```python
from build123d import *

# Parameters (mm, degrees)
SKETCH1_W                                        = 160
SKETCH1_H                                        = 150
BOSS_EXTRUDE1_DEPTH                              = 4.76
F_7_0_7_DIAMETER_HOLE1_D                         = 7
CBORE_FOR_M3_HEX_HEAD_MACHINE_SCREW1_D           = 3.5
CBORE_FOR_M3_HEX_HEAD_MACHINE_SCREW1_CBORE_D     = 6.5
CBORE_FOR_M3_HEX_HEAD_MACHINE_SCREW1_CBORE_DEPTH = 2
F_3_0_3_DIAMETER_HOLE1_D                         = 3
M27_CLEARANCE_HOLE1_D                            = 30


with BuildPart() as part:
    # Sketch1 → Boss-Extrude1 (new body)
    with BuildSketch(Plane.XY.offset(4.76)):
        with Locations((-10, 0)):
            Rectangle(SKETCH1_W, SKETCH1_H)
    extrude(amount=-BOSS_EXTRUDE1_DEPTH)

    # Sketch2 → Cut-Revolve1 (revolve, cut)
    with BuildSketch(Plane(origin=(0, 36.935244785, 0), x_dir=(1, 0, 0), z_dir=(0, 1, 0))):
        Polygon((35.647279442, 0), (34.026279442, 0), (34.026279442, -4.76), (35.647279442, -4.76), (35.647279442, -2.76), align=None)
    revolve(axis=Axis((34.026279442, 36.935244785, 0), (0, 0, 1)), mode=Mode.SUBTRACT)

    # Sketch3 → Cut-Revolve2 (revolve, cut)
    with BuildSketch(Plane(origin=(0, 11, 0), x_dir=(1, 0, 0), z_dir=(0, 1, 0))):
        Polygon((-47.379, 0), (-49, 0), (-49, -4.76), (-47.379, -4.76), (-47.379, -2.76), align=None)
    revolve(axis=Axis((-49, 11, 0), (0, 0, 1)), mode=Mode.SUBTRACT)

    # Sketch4 → Cut-Revolve3 (revolve, cut)
    with BuildSketch(Plane(origin=(0, -36.935244785, 0), x_dir=(1, 0, 0), z_dir=(0, 1, 0))):
        Polygon((35.647279442, 0), (34.026279442, 0), (34.026279442, -4.76), (35.647279442, -4.76), (35.647279442, -2.76), align=None)
    revolve(axis=Axis((34.026279442, -36.935244785, 0), (0, 0, 1)), mode=Mode.SUBTRACT)

    # Sketch5 → Cut-Revolve4 (revolve, cut)
    with BuildSketch(Plane(origin=(0, -47.935244785, 0), x_dir=(1, 0, 0), z_dir=(0, 1, 0))):
        Polygon((16.594720558, 0), (14.973720558, 0), (14.973720558, -4.76), (16.594720558, -4.76), (16.594720558, -2.76), align=None)
    revolve(axis=Axis((14.973720558, -47.935244785, 0), (0, 0, 1)), mode=Mode.SUBTRACT)

    # Sketch6 → Cut-Revolve5 (revolve, cut)
    with BuildSketch(Plane(origin=(0, 47.935244785, 0), x_dir=(1, 0, 0), z_dir=(0, 1, 0))):
        Polygon((16.594720558, 0), (14.973720558, 0), (14.973720558, -4.76), (16.594720558, -4.76), (16.594720558, -2.76), align=None)
    revolve(axis=Axis((14.973720558, 47.935244785, 0), (0, 0, 1)), mode=Mode.SUBTRACT)

    # Sketch7 → Cut-Revolve6 (revolve, cut)
    with BuildSketch(Plane(origin=(0, -11, 0), x_dir=(1, 0, 0), z_dir=(0, 1, 0))):
        Polygon((-47.379, 0), (-49, 0), (-49, -4.76), (-47.379, -4.76), (-47.379, -2.76), align=None)
    revolve(axis=Axis((-49, -11, 0), (0, 0, 1)), mode=Mode.SUBTRACT)

    # Ø7.0 (7) Diameter Hole1 (through all)
    with Locations(Plane(origin=(0, 0, 0), x_dir=(-1, 0, 0), z_dir=(0, 0, -1))):
        with Locations((3, -41.5)):
            Hole(F_7_0_7_DIAMETER_HOLE1_D / 2)

    # CBORE for M3 Hex Head Machine Screw1 (through all)
    with Locations(Plane.XY.offset(4.76)):
        with Locations((-70, -70), (60, -60), (-84.999999999, 54.667182961), (60, 54.667182961), (-84.999999999, -38.000000001)):
            CounterBoreHole(CBORE_FOR_M3_HEX_HEAD_MACHINE_SCREW1_D / 2, CBORE_FOR_M3_HEX_HEAD_MACHINE_SCREW1_CBORE_D / 2, CBORE_FOR_M3_HEX_HEAD_MACHINE_SCREW1_CBORE_DEPTH)

    # Ø3.0 (3) Diameter Hole1 (through all)
    with Locations(Plane(origin=(0, 0, 0), x_dir=(-1, 0, 0), z_dir=(0, 0, -1))):
        with Locations((20.75, 35.940054257), (18.25, 31.609927238), (20.75, -35.940054257), (18.25, -31.609927238), (-41.5, 0), (-29.250000001, 50.662486121), (-26.750000001, 46.332359102), (-36.5, 0), (58.5, 1e-09), (53.5, 1e-09), (-26.749999999, -46.332359103), (-29.249999999, -50.662486122)):
            Hole(F_3_0_3_DIAMETER_HOLE1_D / 2)

    # M27 Clearance Hole1 (through all)
    with Locations(Plane(origin=(0, 0, 0), x_dir=(-1, 0, 0), z_dir=(0, 0, -1))):
        with Locations((0, 0)):
            Hole(M27_CLEARANCE_HOLE1_D / 2)


solid = part.part
```
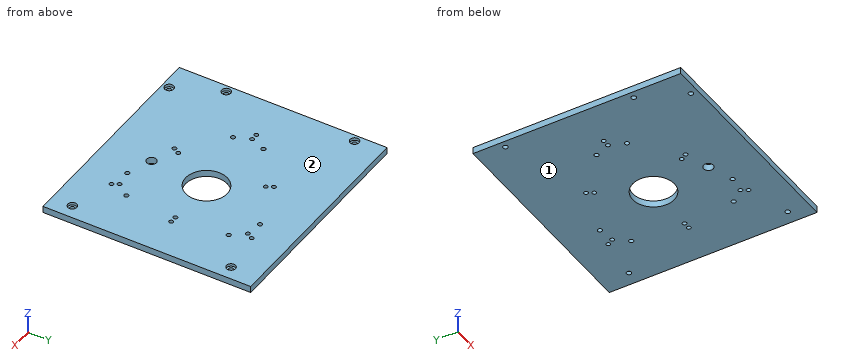
Geometry: final body of the model. Coordinates: model frame, mm. Face numbers are marked on the shaded views. Coordinates: 2 decimals unless noted, no trailing zeros. Order: outer loops, then holes, each group sorted by start corner. A loop starts at its lowest first (then second) coordinate and runs counter-clockwise, first axis right, second up. Notation, with made-up numbers: (-27, 38.5) -> (13, 38.5) arc R15 cw to (13, 52.5) -> close; hole circle Ø1 at (64.25, 89). An arc over 180 degrees is marked (long way). Write item = value, one per line.
(1) Line query: line 1 (Y direction, x = 29.5, z = 2.8); line 2 (Y direction, x = 34.5, z = 0.75) (3 decimals); line 3 (X direction, y = 46, z = 3.45). Output: solid intervals per line, ascending.
Solved:
line_1 = -75 to -52.14, -49.18 to 49.18, 52.14 to 75
line_2 = -75 to -38.485, -35.385 to 35.385, 38.485 to 75
line_3 = -90 to 25.29, 28.21 to 70
(2) Cut plane B-B on z = 3.95. Count the separate pieces of the cut face and the enclosed holes in it, plus the area to 3 significant figures.
Solved:
separate_pieces = 1
enclosed_holes = 25
area = 23,000 mm²
(3) Cut plane A-A on x = -3. Return loops of the section in (y, z).
Solved:
outline = (-75, 0) -> (-45, 0) -> (-45, 4.76) -> (-75, 4.76) -> close; (-38, 0) -> (-14.7, 0) -> (-14.7, 4.76) -> (-38, 4.76) -> close; (14.7, 0) -> (75, 0) -> (75, 4.76) -> (14.7, 4.76) -> close
(4) Pull-direction query (Z, two-part tool) for the marked faces 1 and 2; classes: pulls with the +Z half, pulls with the -Z half, needs draft (parallel to the pull), parting line crosses it, or undercut.
Solved:
face_1 = pulls with the -Z half
face_2 = pulls with the +Z half
(5) Pin query (flat end, axial travel): pin 1 Ø2.5 at (x, y) = (14.97, -47.94) entering from +Z; pin 2 Ø4.5 at (x, y) = (-85, 54.67) entering from +Z. Return the tip coordinate at first contact, or that it passes through.
Solved:
pin_1 = through
pin_2 = 2.76
